from build123d import *

# Parameters (mm, degrees)
F0_W     = 38
F0_H     = 12
F0_R     = 3.6
F1_DEPTH = 10
F2_W     = 16
F2_H     = 4
F3_DEPTH = 12.001
F4_R     = 2


with BuildPart() as f1:
    # F0 (on Top) → F1 (new body)
    with BuildSketch(Plane.XY):
        Rectangle(F0_W, F0_H)
        with Locations((-12.5, 0)):
            Circle(F0_R, mode=Mode.SUBTRACT)
        with Locations((12.5, 0)):
            Circle(F0_R, mode=Mode.SUBTRACT)
    extrude(amount=F1_DEPTH)

    # F2 (on face) → F3 (cut, through all)
    with BuildSketch(Plane.XZ.offset(6)):
        with Locations((0, 2)):
            Rectangle(F2_W, F2_H)
    extrude(amount=-F3_DEPTH, mode=Mode.SUBTRACT)

    # F4
    f4_edges = [f1.edges().sort_by_distance(p)[0] for p in [
        (-8, 0, 4),
        (8, 0, 4),
    ]]
    fillet(f4_edges, radius=F4_R)


solid = f1.part
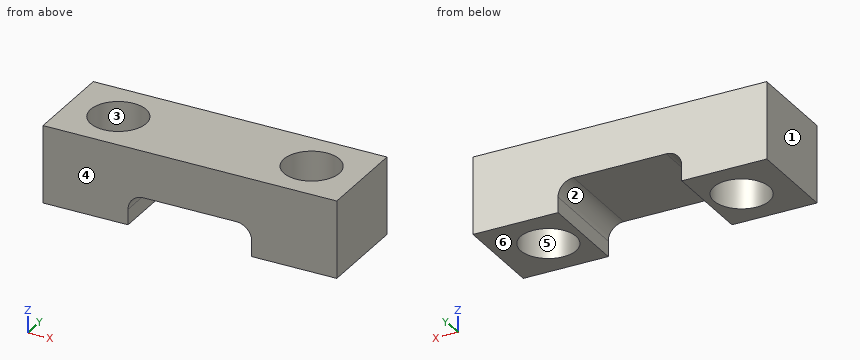
Here's how the part is built. I have some questions about the finished solid (model axes, mm). Face numbers are marked on the shaded views. A direction names the side the tool comes from. Coordinates: 2 decimals unless noted, no trailing zeros. Order: outer loops, then holes, each group sorted by start corner. A loop starts at its lowest first (then second) coordinate and runs counter-clockwise, first axis right, second up. Notation, with made-up numbers: M -10,39.25 L 37,39.25 A26 cw 37,66.25 Z; hole C -8.5,-20 d1. An arc over 180 degrees is marked long. Answer as CSV lines item,"result".
Item 1: Imagine slicing it at C-C on z = 9. Write out the boundary of the cut face in (x, y).
Results found:
outline,"M -19,-6 L 19,-6 L 19,6 L -19,6 Z; hole C -12.5,0 d7.2; hole C 12.5,0 d7.2"
Item 2: We'd pull the mould along Y, two halves only. Please class the marked faces 3, 4, 5 and 6: +Y half, -Y half, draft (parallel to the pull), parting line (faces both ways), or undercut.
Results found:
face 3,"undercut"
face 4,"-Y half"
face 5,"undercut"
face 6,"draft"
Item 3: On a 3-axis mill with a long thin cutter (end or side, diameter ignored), from which of +Z, -Z, +X, -X, +Y, -Y can I reach the whole of each face in a straight line? I mean the marked faces 1 and 2. Say none if no direction works.
Results found:
face 1,"+Z, -Z, -X, +Y, -Y"
face 2,"-Z, +Y, -Y"
Item 4: Imagine slicing it at D-D on y = 5.25. Write out the boundary of the cut face in (x, z).
Results found:
outline,"M -19,0 L -8,0 L -8,2 A2 cw -6,4 L 6,4 A2 cw 8,2 L 8,0 L 19,0 L 19,10 L -19,10 Z"
Item 5: If I drill on line 1 (Y direction, x = -12.5, z = 6.5); line 2 (X direction, y = -3.25, z = 4.25); line 3 (X direction, y = 1.5, z = 6.5), over which ranges is the centre line in solid material (lowest first)?
Results found:
line 1,"-6 to -3.6, 3.6 to 6"
line 2,"-19 to -14.05, -10.95 to 10.95, 14.05 to 19"
line 3,"-19 to -15.77, -9.23 to 9.23, 15.77 to 19"
Item 6: For pin 1 (4 mm diameter, centred on x = -11.5, y = -1, fed in from +Z); pin 2 (6 mm diameter, centred on x = -2, y = 0, fed in from -Z), each with a flat end and sliding along its axis, tell me the tip position at first contact or that it passes through.
Results found:
pin 1,"through"
pin 2,"z = 4"
Item 7: Imagine slicing it at A-A on x = -12.5. Write out the boundary of the cut face in (y, z).
Results found:
outline,"M -6,0 L -3.6,0 L -3.6,10 L -6,10 Z; M 3.6,0 L 6,0 L 6,10 L 3.6,10 Z"
Item 8: Imagine slicing it at B-B on y = 0. Write out the boundary of the cut face in (x, z).
Results found:
outline,"M -19,0 L -16.1,0 L -16.1,10 L -19,10 Z; M -8.9,0 L -8,0 L -8,2 A2 cw -6,4 L 6,4 A2 cw 8,2 L 8,0 L 8.9,0 L 8.9,10 L -8.9,10 Z; M 16.1,0 L 19,0 L 19,10 L 16.1,10 Z"
